from build123d import *

# Parameters (mm, degrees)
SKETCH1_W           = 31
SKETCH1_H           = 62
BOSS_EXTRUDE1_DEPTH = 9
SKETCH2_R           = 2
CUT_EXTRUDE1_DEPTH  = 10
SKETCH3_R           = 3.5
CUT_EXTRUDE2_DEPTH  = 4


with BuildPart() as part:
    # Sketch1 → Boss-Extrude1 (new body)
    with BuildSketch(Plane.XY):
        Rectangle(SKETCH1_W, SKETCH1_H)
    extrude(amount=BOSS_EXTRUDE1_DEPTH)

    # Sketch2 → Cut-Extrude1 (cut)
    with BuildSketch(Plane.XY.offset(9)):
        with Locations((0, 27)):
            Circle(SKETCH2_R)
        with Locations((0, -27)):
            Circle(SKETCH2_R)
        with Locations((10.5, 0)):
            Circle(SKETCH2_R)
        with Locations((-10.5, 0)):
            Circle(SKETCH2_R)
    extrude(amount=-CUT_EXTRUDE1_DEPTH, mode=Mode.SUBTRACT)

    # Sketch3 → Cut-Extrude2 (cut)
    with BuildSketch(Plane.XY.offset(9)):
        with Locations((0, 27)):
            Circle(SKETCH3_R)
        with Locations((10.5, 0)):
            Circle(SKETCH3_R)
        with Locations(Location((-10.5, 0, 0), (0, 0, 180))):
            Circle(SKETCH3_R)
        with Locations(Location((0, -27, 0), (0, 0, 180))):
            Circle(SKETCH3_R)
    extrude(amount=-CUT_EXTRUDE2_DEPTH, mode=Mode.SUBTRACT)


solid = part.part
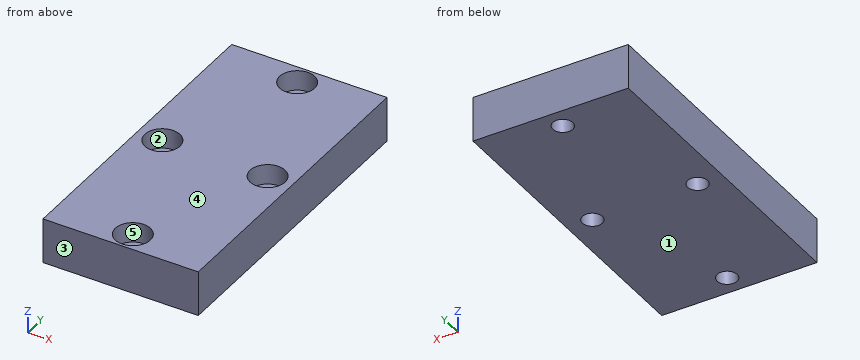
Build history of the part. All positions in model axes, mm. Face numbers are marked on the shaded views. A direction names the side the tool comes from. Round coordinates to 2 decimals unless told otherwise and drop trailing zeros. Write each loop counter-clockwise with the first axis right and the second up, starting at its lowest first coordinate (ties: lowest second). Pieces come first, ordered by that corner, then holes. Notation, with made-up numbers: (19, 2.5) - (75, 2.5) arc R25 cw to (75, 40.5) - close; hole circle Ø8 at (-14.75, 38). An arc over 180 degrees is marked (long way). Use CSV: the item, a comma, the result in double quotes.
(1) Band-saw the part on C-C (y = 0). Write the cut outline in (x, z), plus the area to 3 significant figures.
Response:
outline,"(-15.5, 0) - (-12.5, 0) - (-12.5, 5) - (-14, 5) - (-14, 9) - (-15.5, 9) - close; (-8.5, 0) - (8.5, 0) - (8.5, 5) - (7, 5) - (7, 9) - (-7, 9) - (-7, 5) - (-8.5, 5) - close; (12.5, 0) - (15.5, 0) - (15.5, 9) - (14, 9) - (14, 5) - (12.5, 5) - close"
area,"183 mm²"
(2) Band-saw the part on A-A (x = -10.5). Write the cut outline in (y, z), plus the area to 3 significant figures.
Response:
outline,"(-31, 0) - (-2, 0) - (-2, 5) - (-3.5, 5) - (-3.5, 9) - (-31, 9) - close; (2, 0) - (31, 0) - (31, 9) - (3.5, 9) - (3.5, 5) - (2, 5) - close"
area,"510 mm²"
(3) 3-axis set-ups, long thin cutter, end or side, ignore diameter. For the marked faces 1 and 2: which of +Z, -Z, +X, -X, +Y, -Y reach the whole face in a straight line?
Response:
face 1,"-Z, +X, -X, +Y, -Y"
face 2,"+Z"
(4) Mould opens along Y. For the marked faces 3, 4 and 5 say: pulls with the +Y half, pulls with the -Y half, needs draft (parallel to the pull), parting line crosses it, or undercut.
Response:
face 3,"pulls with the -Y half"
face 4,"needs draft"
face 5,"undercut"
(5) Wall check: line 1 (Y direction, x = 0, z = 2.85); line 2 (X direction, y = -0.5, z = 5.5); line 3 (Y direction, x = 10.5, z = 8.15). Give the ranges that are in metal, low to high.
Response:
line 1,"-31 to -29, -25 to 25, 29 to 31"
line 2,"-15.5 to -13.96, -7.04 to 7.04, 13.96 to 15.5"
line 3,"-31 to -3.5, 3.5 to 31"
(6) Band-saw the part on B-B (y = 27). Write the cut outline in (x, z), plus the area to 3 significant figures.
Response:
outline,"(-15.5, 0) - (-2, 0) - (-2, 5) - (-3.5, 5) - (-3.5, 9) - (-15.5, 9) - close; (2, 0) - (15.5, 0) - (15.5, 9) - (3.5, 9) - (3.5, 5) - (2, 5) - close"
area,"231 mm²"
(7) Band-saw the part on D-D (z = 2.25). Write the cut outline in (x, y).
Response:
outline,"(-15.5, -31) - (15.5, -31) - (15.5, 31) - (-15.5, 31) - close; hole circle Ø4 at (-10.5, 0); hole circle Ø4 at (0, -27); hole circle Ø4 at (0, 27); hole circle Ø4 at (10.5, 0)"
(8) Pin check, flat tips, straight feed: P1, Ø8, axis at x = 0, y = 27, coming from the +Z side; P2, Ø5.5, axis at x = -10.5, y = 0, coming from the +Z side; P3, Ø3.5, axis at x = 10.5, y = 0, coming from the +Z side. Stop position of each tip, or through.
Response:
P1,"z = 9"
P2,"z = 5"
P3,"through"
